```python
from build123d import *

# Parameters (mm, degrees)
SKETCH1_W             = 2.412698413
SKETCH1_H             = 44
BOSS_EXTRUDE1_DEPTH   = 10
SKETCH1_W_2           = 4.015873015
BOSS_EXTRUDE1_2_DEPTH = 10
SKETCH1_W_3           = 4.19047619
BOSS_EXTRUDE1_3_DEPTH = 10
SKETCH1_W_4           = 3.80952381
BOSS_EXTRUDE1_4_DEPTH = 10
SKETCH1_W_5           = 3.841269842
BOSS_EXTRUDE1_5_DEPTH = 10
SKETCH2_R             = 1.633949522
SKETCH2_R_2           = 1.683053635
SKETCH2_R_3           = 1.598900953
SKETCH2_R_4           = 1.514748271
SKETCH2_R_5           = 1.767206317
SKETCH2_R_6           = 1.734851978
SKETCH2_R_7           = 1.920820677
BOSS_EXTRUDE2_DEPTH   = 79
SKETCH3_W             = 3.415155575
SKETCH3_H             = 9.375258814
CUT_EXTRUDE1_DEPTH    = 43
SKETCH4_W             = 3.285780113
SKETCH4_H             = 9.121325595
CUT_EXTRUDE2_DEPTH    = 43
SKETCH5_W             = 3.071339727
SKETCH5_H             = 9.276276067
CUT_EXTRUDE3_DEPTH    = 43
SKETCH6_W             = 3.446725694
SKETCH6_H             = 9.487027157
CUT_EXTRUDE4_DEPTH    = 43
SKETCH7_W             = 1.989906413
SKETCH7_H             = 9.551550778
CUT_EXTRUDE5_DEPTH    = 43
SKETCH8_W             = 82
SKETCH8_H             = 10
BOSS_EXTRUDE3_DEPTH   = 0.2


with BuildPart() as part:
    # Sketch1 → Boss-Extrude1 (new body)
    with BuildSketch(Plane.XY):
        with Locations((-39.793650793, 0)):
            Rectangle(SKETCH1_W, SKETCH1_H)
    extrude(amount=BOSS_EXTRUDE1_DEPTH)



with BuildPart() as body_2:
    # Sketch1 → Boss-Extrude1 2 (new body)
    with BuildSketch(Plane.XY):
        with Locations((-24.182539682, 0)):
            Rectangle(SKETCH1_W_2, SKETCH1_H)
    extrude(amount=BOSS_EXTRUDE1_2_DEPTH)


with BuildPart() as body_3:
    # Sketch1 → Boss-Extrude1 3 (new body)
    with BuildSketch(Plane.XY):
        with Locations((17.984126984, 0)):
            Rectangle(SKETCH1_W_3, SKETCH1_H)
    extrude(amount=BOSS_EXTRUDE1_3_DEPTH)


with BuildPart() as body_4:
    # Sketch1 → Boss-Extrude1 4 (new body)
    with BuildSketch(Plane.XY):
        with Locations((39.095238095, 0)):
            Rectangle(SKETCH1_W_4, SKETCH1_H)
    extrude(amount=BOSS_EXTRUDE1_4_DEPTH)


with BuildPart() as body_5:
    # Sketch1 → Boss-Extrude1 5 (new body)
    with BuildSketch(Plane.XY):
        Rectangle(SKETCH1_W_5, SKETCH1_H)
    extrude(amount=BOSS_EXTRUDE1_5_DEPTH)


with BuildPart() as part_1:
    add(part.part)

    add(body_2.part)  # Boss-Extrude2 merges body 2

    add(body_3.part)  # Boss-Extrude2 merges body 3

    add(body_4.part)  # Boss-Extrude2 merges body 4

    add(body_5.part)  # Boss-Extrude2 merges body 5
    # Sketch2 → Boss-Extrude2 (add)
    with BuildSketch(Plane(origin=(-38.587301587, 0, 0), x_dir=(0, 0, -1), z_dir=(1, 0, 0))):
        with Locations(Location((-5.420903309, 19.425806282, 0), (0, 0, 180))):
            Circle(SKETCH2_R)
        with Locations(Location((-5.420903309, 13.450965878, 0), (0, 0, 180))):
            Circle(SKETCH2_R_2)
        with Locations(Location((-5.420903309, 7.896888883, 0), (0, 0, 180))):
            Circle(SKETCH2_R_3)
        with Locations(Location((-5.420903309, 2.090353843, 0), (0, 0, 180))):
            Circle(SKETCH2_R_2)
        with Locations(Location((-5.420903309, -3.632028516, 0), (0, 0, 180))):
            Circle(SKETCH2_R_4)
        with Locations(Location((-5.420903309, -10.027632329, 0), (0, 0, 180))):
            Circle(SKETCH2_R_5)
        with Locations(Location((-5.420903309, -15.160945915, 0), (0, 0, 180))):
            Circle(SKETCH2_R_6)
        with Locations(Location((-5.420903309, -19.452732684, 0), (0, 0, 180))):
            Circle(SKETCH2_R_7)
    extrude(amount=BOSS_EXTRUDE2_DEPTH)

    # Sketch3 → Cut-Extrude1 (cut)
    with BuildSketch(Plane.XZ.offset(22)):
        with Locations((39.124547019, 4.970791564)):
            Rectangle(SKETCH3_W, SKETCH3_H)
    extrude(amount=-CUT_EXTRUDE1_DEPTH, mode=Mode.SUBTRACT)

    # Sketch4 → Cut-Extrude2 (cut)
    with BuildSketch(Plane.XZ.offset(22)):
        with Locations((17.868418128, 5.008563078)):
            Rectangle(SKETCH4_W, SKETCH4_H)
    extrude(amount=-CUT_EXTRUDE2_DEPTH, mode=Mode.SUBTRACT)

    # Sketch5 → Cut-Extrude3 (cut)
    with BuildSketch(Plane.XZ.offset(22)):
        with Locations((-0.004150459, 4.964721098)):
            Rectangle(SKETCH5_W, SKETCH5_H)
    extrude(amount=-CUT_EXTRUDE3_DEPTH, mode=Mode.SUBTRACT)

    # Sketch6 → Cut-Extrude4 (cut)
    with BuildSketch(Plane.XZ.offset(22)):
        with Locations((-24.197176497, 4.985015311)):
            Rectangle(SKETCH6_W, SKETCH6_H)
    extrude(amount=-CUT_EXTRUDE4_DEPTH, mode=Mode.SUBTRACT)

    # Sketch7 → Cut-Extrude5 (cut)
    with BuildSketch(Plane.XZ.offset(22)):
        with Locations((-39.773791775, 5.027285399)):
            Rectangle(SKETCH7_W, SKETCH7_H)
    extrude(amount=-CUT_EXTRUDE5_DEPTH, mode=Mode.SUBTRACT)

    # Sketch8 → Boss-Extrude3 (add)
    with BuildSketch(Plane.XZ.offset(22)):
        with Locations((0, 5)):
            Rectangle(SKETCH8_W, SKETCH8_H)
    extrude(amount=BOSS_EXTRUDE3_DEPTH)


solid = part_1.part
```
Work out the finished part from the listing and answer in its coordinate system (mm). A direction names the side the tool comes from. Round coordinates to 2 decimals unless told otherwise and drop trailing zeros. Write each question's results on one line, items separated by ' | '. Start each with the question number.
1. A tool of negligible diameter and unlimited length cuts with its end or side. For faces 4 (the face through (29, -22, 5)), 5 (the face through (8.81, -17.58, 5)), from which of +Z, -Z, +X, -X, +Y, -Y can it reach the whole face along a straight path? Write none if from no direction.
2. Given pin 1 Ø1.5 at (x, y) = (-12, 16.5) entering from -Z; pin 2 Ø3 at (x, z) = (-8, 6) entering from +Y; pin 3 Ø3 at (x, y) = (30.5, -12) entering from -Z, each flat-ended and moving along its own axis, determine where each tip first touches the part or whether it passes through.
3. For a pull along Z with two mould halves and no side action, classify faces 1 (the face through (-12.2, -11.2, 4.1)), 2 (the face through (-24, -22, 5)), 3 (the face through (41, 0, 5)) as +Z half, -Z half, draft (parallel to the pull), parting line (faces both ways), or undercut.
4. Find the intervals of material crossed by probe 1 along X at (y, z) = (2.5, 4.25); probe 2 along Y at (x, z) = (37.5, 2.25); probe 3 along Z at (x, y) = (6, -10), in increasing order. Write a range as from..to.
5. Section A-A (y = -6) is taken. State how many separate pieces and enclosed holes the cut face has, plus the area to 3 significant figures.
Evaluation:
1) face 4: +Z, -Z | face 5: none
2) pin 1: passes through | pin 2: stops at y = 21.06 | pin 3: stops at z = 3.72
3) face 1: parting line | face 2: undercut | face 3: draft
4) probe 1: x = -41..-40.77, -38.78..-25.92, -22.47..-1.54, 1.53..16.23, 19.51..37.42, 40.83..41 | probe 2: y = -22.2..-22, 21..22 | probe 3: z = 3.65..7.19
5) separate pieces: 5 | enclosed holes: 5 | area: 40.5 mm2
